The listing builds one solid part. Answer for the finished solid, in the listing's coordinates (mm). A direction names the side the tool comes from. Coordinates: 2 decimals unless noted, no trailing zeros. Loops run counter-clockwise (first coordinate to the right, second up) from the corner with the lowest first, then second, coordinate; pieces in that order, holes last. Notation, with made-up numbers: (75, 17) -> (116, 17) arc R20 cw to (116, 50) -> close; hole circle Ø4 at (-29, 58). An arc over 180 degrees is marked (long way). Answer in a Markdown table with one row per item.
```python
from build123d import *

# Parameters (mm, degrees)
BOSS_EXTRUDE1_DEPTH = 3
CUT_EXTRUDE1_DEPTH  = 10
LPATTERN1_COUNT     = 6
LPATTERN1_PITCH     = 25
CUT_EXTRUDE2_DEPTH  = 10
LPATTERN2_COUNT     = 6
LPATTERN2_PITCH     = 25
CAVITY1_START       = 77
CAVITY1_OUTLINE_W   = 15
CAVITY1_OUTLINE_H   = 3
CAVITY1_OUTLINE_W_2 = 10
CAVITY1_OUTLINE_W_3 = 25
CAVITY1_DEPTH       = 3
SKETCH5_W           = 60
SKETCH5_H           = 50
CUT_EXTRUDE3_DEPTH  = 10
FILLET1_R           = 10


# Read off the part's stored shape, not the designer's step: Cavity1
with BuildPart() as part:
    # Sketch1 → Boss-Extrude1 (new body)
    with BuildSketch(Plane.XY):
        Polygon((-170, -80), (170, -80), (90, 80), (-90, 80), align=None)
    extrude(amount=BOSS_EXTRUDE1_DEPTH)

    # Sketch2 → Cut-Extrude1 (cut)
    with BuildSketch(Plane.XY.offset(3)):
        Polygon((-158.819660113, -57.639320225), (-152.11145618, -44.22291236), (-149.428174607, -45.564553147), (-156.13637854, -58.980961012), align=None)
    cut_extrude1 = extrude(amount=-CUT_EXTRUDE1_DEPTH, mode=Mode.SUBTRACT)

    # LPattern1: Cut-Extrude1 ×6
    with Locations(*[Vector(0.44721359549995776, 0.894427190999916, 0) * (i * LPATTERN1_PITCH) for i in range(1, LPATTERN1_COUNT)]):
        add(cut_extrude1, mode=Mode.SUBTRACT)

    # Sketch3 → Cut-Extrude2 (cut)
    with BuildSketch(Plane.XY.offset(3)):
        Polygon((158.819660113, -57.639320225), (152.11145618, -44.22291236), (149.428174607, -45.564553147), (156.13637854, -58.980961012), align=None)
    cut_extrude2 = extrude(amount=-CUT_EXTRUDE2_DEPTH, mode=Mode.SUBTRACT)

    # LPattern2: Cut-Extrude2 ×6
    with Locations(*[Vector(-0.4472135954999582, 0.8944271909999159, 0) * (i * LPATTERN2_PITCH) for i in range(1, LPATTERN2_COUNT)]):
        add(cut_extrude2, mode=Mode.SUBTRACT)

    # Cavity1 outline → Cavity1 (cut)
    with BuildSketch(Plane(origin=(0, 0, 0), x_dir=(1, 0, 0), z_dir=(0, 1, 0)).offset(CAVITY1_START)):
        with Locations((-82.5, -1.5)):
            Rectangle(CAVITY1_OUTLINE_W, CAVITY1_OUTLINE_H)
        with Locations((-55, -1.5)):
            Rectangle(CAVITY1_OUTLINE_W_2, CAVITY1_OUTLINE_H)
        with Locations((-30, -1.5)):
            Rectangle(CAVITY1_OUTLINE_W_2, CAVITY1_OUTLINE_H)
        with Locations((-5, -1.5)):
            Rectangle(CAVITY1_OUTLINE_W_2, CAVITY1_OUTLINE_H)
        with Locations((20, -1.5)):
            Rectangle(CAVITY1_OUTLINE_W_2, CAVITY1_OUTLINE_H)
        with Locations((45, -1.5)):
            Rectangle(CAVITY1_OUTLINE_W_2, CAVITY1_OUTLINE_H)
        with Locations((77.5, -1.5)):
            Rectangle(CAVITY1_OUTLINE_W_3, CAVITY1_OUTLINE_H)
    extrude(amount=CAVITY1_DEPTH, mode=Mode.SUBTRACT)

    # Sketch5 → Cut-Extrude3 (cut)
    with BuildSketch(Plane.XY.offset(3)):
        with Locations((0, 11.03685601)):
            Rectangle(SKETCH5_W, SKETCH5_H)
    extrude(amount=-CUT_EXTRUDE3_DEPTH, mode=Mode.SUBTRACT)

    # Fillet1
    fillet1_edges = [part.edges().sort_by_distance(p)[0] for p in [
        (30, 36.03685601, 1.5),
        (30, -13.96314399, 1.5),
        (-30, -13.96314399, 1.5),
        (-30, 36.03685601, 1.5),
    ]]
    fillet(fillet1_edges, radius=FILLET1_R)


solid = part.part
```
Item 1: Flat-ended cylindrical pins translate along their axes: pin 1 Ø0.9 at (x, z) = (78.5, 2) entering from +Y; pin 2 Ø1.5 at (y, z) = (79, 2) entering from +X (3 decimals); pin 3 Ø1.5 at (y, z) = (78.5, 1.5) entering from -X (3 decimals). Find the tip coordinate at first contact, or state that the pin passes through.
Findings below:
| item | result |
|---|---|
| pin 1 | stops at y = 77 |
| pin 2 | stops at x = 90.875 |
| pin 3 | stops at x = -91.125 |
Item 2: Find the intervals of material crossed by probe 1 along Y at (x, z) = (-5.5, 1.85); probe 2 along Y at (x, z) = (-15.5, 0.55); probe 3 along Y at (x, z) = (85, 2.8), in increasing order.
Findings below:
| item | result |
|---|---|
| probe 1 | y = -80 to -13.96, 36.04 to 77 |
| probe 2 | y = -80 to -13.96, 36.04 to 80 |
| probe 3 | y = -80 to 77 |
Item 3: Determine the mould class of faces 1 (the face through (-2, -17, 0)), 2 (the face through (26.993, -11.112, 1.479)), 3 (the face through (-26.993, -11.112, 1.479)), 4 (the face through (-93, 74, 1)) for opening direction X: +X half, -X half, draft (parallel to the pull), parting line (faces both ways), or undercut.
Findings below:
| item | result |
|---|---|
| face 1 | draft |
| face 2 | undercut |
| face 3 | undercut |
| face 4 | -X half |
Item 4: A cutting plane is placed at A-A, the plane x = 82. Determine the outline of the cut face in (y, z), plus the area to 3 significant figures.
Findings below:
| item | result |
|---|---|
| outline | (-80, 0) -> (77, 0) -> (77, 3) -> (-80, 3) -> close |
| area | 471 mm2 |
Item 5: A cutting plane is placed at B-B, the plane y = -64. Determine the outline of the cut face in (x, z).
Findings below:
| item | result |
|---|---|
| outline | (-162, 0) -> (162, 0) -> (162, 3) -> (-162, 3) -> close |
Item 6: A tool of negligible diameter and unlimited length cuts with its end or side. For faces 5 (the face through (-26.99, 33.19, 1.48)), 6 (the face through (93, 74, 1)), from which of +Z, -Z, +X, -X, +Y, -Y can it reach the whole face along a straight path? Write none if from no direction.
Findings below:
| item | result |
|---|---|
| face 5 | +Z, -Z |
| face 6 | +Z, -Z, +X, +Y |
